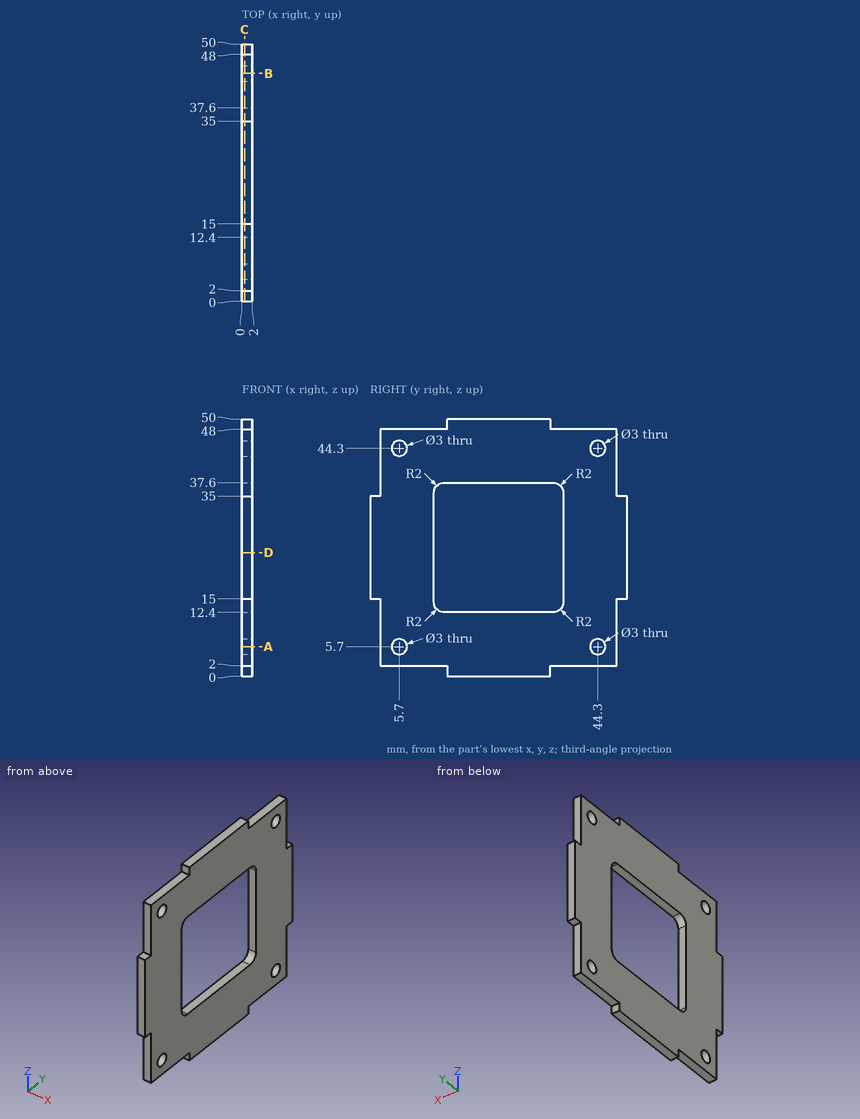
Study the drawing (mm; zero at the part's minimum x, y, z) and answer. Give positions to 0.01 mm unless a question says otherwise; leave off trailing zeros. Write each loop counter-clockwise with the first axis right and the second up, starting at its lowest first coordinate (ties: lowest second). Pieces come first, ordered by that corner, then holes. Notation, with made-up numbers: (77, 52) -> (124, 52) arc R36 ccw to (124, 90) -> close; hole circle Ø5 at (38.5, 27.25). An arc over 180 degrees is marked (long way). Write item = value, one per line. Start each with the question number.
1) Each of these flat-tipped pins is pushed along its axis until it touches: pin 1 (1 mm diameter, centred on x = 1, z = 49, fed in from +Y); pin 2 (1 mm diameter, centred on x = 0.5, z = 16.5, fed in from -Y); pin 3 (1 mm diameter, centred on y = 13, z = 24, fed in from +X); pin 4 (0.6 mm diameter, centred on x = 1, z = 42.5, fed in from +Y). Where does it stop, or does it pass through?
2) The part is cut by section A-A, the plane z = 5.7. Determine the outline of the cut face in (x, y).
3) The part is cut by section C-C, the plane x = 0.55. Count the separate pieces of the cut face and the enclosed holes in it, and give its area (3 significant figures).
4) The part is cut by section D-D, the plane z = 24. Determine the outline of the cut face in (x, y).
5) Straight lines are drawn through the part: line 1 along Z through (x, y) = (1.4, 44.3); line 2 along Z through (x, y) = (1.55, 6.5). For each, find the intervals that lie inside material, in ascending order.
Solutions:
q1.pin_1 = 35
q1.pin_2 = 0
q1.pin_3 = through
q1.pin_4 = 48
q2.outline = (0, 2) -> (2, 2) -> (2, 4.2) -> (0, 4.2) -> close; (0, 7.2) -> (2, 7.2) -> (2, 42.8) -> (0, 42.8) -> close; (0, 45.8) -> (2, 45.8) -> (2, 48) -> (0, 48) -> close
q3.separate_pieces = 1
q3.enclosed_holes = 5
q3.area = 1,620 mm²
q4.outline = (0, 0) -> (2, 0) -> (2, 12.4) -> (0, 12.4) -> close; (0, 37.6) -> (2, 37.6) -> (2, 50) -> (0, 50) -> close
q5.line_1 = 2 to 4.2, 7.2 to 42.8, 45.8 to 48
q5.line_2 = 2 to 4.43, 6.97 to 43.03, 45.57 to 48
